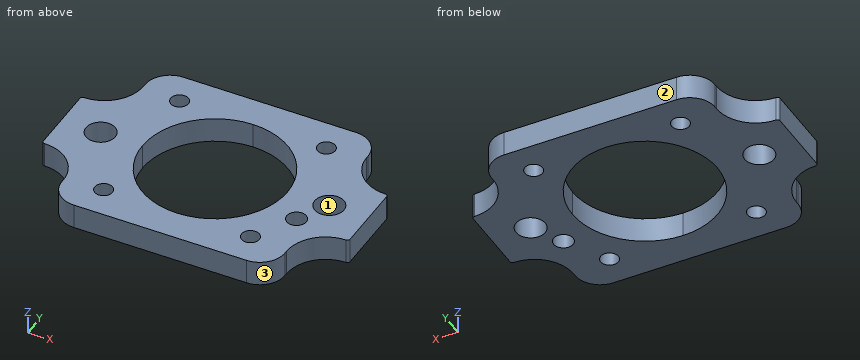
```python
from build123d import *

# Parameters (mm, degrees)
F0_R     = 3.175
F0_R_2   = 6
F0_R_3   = 3.5
F1_DEPTH = 9


with BuildPart() as f1:
    # F0 (on Top) → F1 (new body)
    with BuildSketch(Plane.XY):
        with BuildLine():
            Line((0, 26), (0, 37.5))
            Line((0, 37.5), (-31, 37.5))
            ThreePointArc((-31, 37.5), (-37.363961, 34.863961), (-40, 28.5))
            Line((-40, 28.5), (-40, 27.5))
            ThreePointArc((-40, 27.5), (-44.100505, 17.600505), (-54, 13.5))
            ThreePointArc((-54, 13.5), (-54.707107, 13.207107), (-55, 12.5))
            Line((-55, 12.5), (-55, 0))
            Line((-55, 0), (-46.25, 0))
            ThreePointArc((-46.25, 0), (-41, 5.25), (-35.75, 0))
            Line((-35.75, 0), (-26, 0))
            ThreePointArc((-26, 0), (-18.384776, 18.384776), (0, 26))
        make_face()
        with Locations((-26.324893, 26)):
            Circle(F0_R, mode=Mode.SUBTRACT)
        with BuildLine():
            Line((31, 37.5), (0, 37.5))
            Line((0, 37.5), (0, 26))
            ThreePointArc((0, 26), (18.384776, 18.384776), (26, 0))
            Line((26, 0), (35.75, 0))
            ThreePointArc((35.75, 0), (41, 5.25), (46.25, 0))
            Line((46.25, 0), (55, 0))
            Line((55, 0), (55, 12.5))
            ThreePointArc((55, 12.5), (54.707107, 13.207107), (54, 13.5))
            ThreePointArc((54, 13.5), (44.100505, 17.600505), (40, 27.5))
            Line((40, 27.5), (40, 28.5))
            ThreePointArc((40, 28.5), (37.363961, 34.863961), (31, 37.5))
        make_face()
        with Locations((26.324893, 26)):
            Circle(F0_R, mode=Mode.SUBTRACT)
        with BuildLine():
            ThreePointArc((0, -26), (-18.384776, -18.384776), (-26, 0))
            Line((-26, 0), (-35.75, 0))
            ThreePointArc((-35.75, 0), (-41, -5.25), (-46.25, 0))
            Line((-46.25, 0), (-55, 0))
            Line((-55, 0), (-55, -12.5))
            ThreePointArc((-55, -12.5), (-54.707107, -13.207107), (-54, -13.5))
            ThreePointArc((-54, -13.5), (-44.100505, -17.600505), (-40, -27.5))
            Line((-40, -27.5), (-40, -28.5))
            ThreePointArc((-40, -28.5), (-37.363961, -34.863961), (-31, -37.5))
            Line((-31, -37.5), (0, -37.5))
            Line((0, -37.5), (0, -26))
        make_face()
        with Locations((-26.324893, -26)):
            Circle(F0_R, mode=Mode.SUBTRACT)
        with BuildLine():
            Line((35.75, 0), (26, 0))
            ThreePointArc((26, 0), (18.384776, -18.384776), (0, -26))
            Line((0, -26), (0, -37.5))
            Line((0, -37.5), (31, -37.5))
            ThreePointArc((31, -37.5), (37.363961, -34.863961), (40, -28.5))
            Line((40, -28.5), (40, -27.5))
            ThreePointArc((40, -27.5), (44.100505, -17.600505), (54, -13.5))
            ThreePointArc((54, -13.5), (54.707107, -13.207107), (55, -12.5))
            Line((55, -12.5), (55, 0))
            Line((55, 0), (46.25, 0))
            ThreePointArc((46.25, 0), (41, -5.25), (35.75, 0))
        make_face()
        with Locations((26.324893, -26)):
            Circle(F0_R, mode=Mode.SUBTRACT)
        with Locations((35, -11)):
            Circle(F0_R_2, mode=Mode.SUBTRACT)
        with Locations((35, -11)):
            Circle(F0_R_2)
        with Locations((35, -11)):
            Circle(F0_R_3, mode=Mode.SUBTRACT)
    extrude(amount=F1_DEPTH)


solid = f1.part
```
CAD build for the part. Positions are in the model's coordinates, mm. Face numbers are marked on the shaded views. Round coordinates to 2 decimals unless told otherwise and drop trailing zeros. Loops run counter-clockwise (first coordinate to the right, second up) from the corner with the lowest first, then second, coordinate; pieces in that order, holes last. Notation, with made-up numbers: M 74,54 L 104,54 A25 ccw 104,75 Z; hole C -38,76.25 d11. An arc over 180 degrees is marked long. Use a Markdown table: item, result. Add a question column.
(1) Cut at D-D (y = -24). Give the cut face in (x, z), and give its area (3 significant figures).
(2) Drill centre lines: line 1 (X direction, y = 3, z = 3); line 2 (Y direction, x = 11.5, z = 2.25); line 3 (Y direction, x = -12.5, z = 5.25). Where is each one in solid material? Low to high.
(3) Flat gauge pins, fed straight in: pin 1 (5 mm diameter, centred on y = -27, z = 3, fed in from -X); pin 2 (0.8 mm diameter, centred on y = -28, z = 6.5, fed in from +X); pin 3 (0.8 mm diameter, centred on y = 28, z = 5, fed in from -X). Where does each tip first touch, or does it go through?
(4) Pull direction Y, two halves, no side cores. Call the marked faces 1, 2 and 3: +Y half, -Y half, draft (parallel to the pull), parting line (faces both ways), or undercut.
(5) Cut at B-B (z = 6). State how many separate pieces and enclosed holes the cut face has, and give its area (3 significant figures).
(6) Cut at C-C (x = 7). Give the cut face in (y, z), and give its area (3 significant figures).
(7) Cut at A-A (y = 8.5). Give the cut face in (x, z), and give its area (3 significant figures).
Geometry says:
| question | item | result |
|---|---|---|
| 1 | outline | M -40.44,0 L -28.79,0 L -28.79,9 L -40.44,9 Z; M -23.86,0 L -10,0 L -10,9 L -23.86,9 Z; M 10,0 L 23.86,0 L 23.86,9 L 10,9 Z; M 28.79,0 L 40.44,0 L 40.44,9 L 28.79,9 Z |
| 1 | area | 459 mm² |
| 2 | line 1 | x = -55 to -45.31, -36.69 to -25.83, 25.83 to 36.69, 45.31 to 55 |
| 2 | line 2 | y = -37.5 to -23.32, 23.32 to 37.5 |
| 2 | line 3 | y = -37.5 to -22.8, 22.8 to 37.5 |
| 3 | pin 1 | stops at x = -40.33 |
| 3 | pin 2 | stops at x = 40 |
| 3 | pin 3 | stops at x = -40 |
| 4 | face 1 | undercut |
| 4 | face 2 | +Y half |
| 4 | face 3 | -Y half |
| 5 | separate pieces | 1 |
| 5 | enclosed holes | 8 |
| 5 | area | 4,450 mm² |
| 6 | outline | M -37.5,0 L -25.04,0 L -25.04,9 L -37.5,9 Z; M 25.04,0 L 37.5,0 L 37.5,9 L 25.04,9 Z |
| 6 | area | 224 mm² |
| 7 | outline | M -55,0 L -24.57,0 L -24.57,9 L -55,9 Z; M 24.57,0 L 55,0 L 55,9 L 24.57,9 Z |
| 7 | area | 548 mm² |
